from build123d import *

# Parameters (mm, degrees)
SKETCH1_W           = 68
SKETCH1_H           = 68
BOSS_EXTRUDE1_DEPTH = 10
SKETCH4_W           = 68
SKETCH4_H           = 68
SKETCH4_W_2         = 30
SKETCH4_H_2         = 30
BOSS_EXTRUDE3_DEPTH = 12
FILLET2_R           = 3
FILLET3_R           = 3
SKETCH5_R           = 3.25
CUT_EXTRUDE2_DEPTH  = 20
CHAMFER1_SIZE       = 3
CHAMFER2_SIZE       = 3


with BuildPart() as part:
    # Sketch1 → Boss-Extrude1 (new body)
    with BuildSketch(Plane(origin=(0, 0, 0), x_dir=(1, 0, 0), z_dir=(0, 1, 0))):
        Rectangle(SKETCH1_W, SKETCH1_H)
    extrude(amount=BOSS_EXTRUDE1_DEPTH)

    # Sketch4 → Boss-Extrude3 (add)
    with BuildSketch(Plane.XZ):
        Rectangle(SKETCH4_W, SKETCH4_H)
        Rectangle(SKETCH4_W_2, SKETCH4_H_2, mode=Mode.SUBTRACT)
    extrude(amount=BOSS_EXTRUDE3_DEPTH)

    # Fillet2
    fillet2_edges = [part.edges().sort_by_distance(p)[0] for p in [
        (34, -1, 34),
        (-34, -1, 34),
        (-34, -1, -34),
        (34, -1, -34),
    ]]
    fillet(fillet2_edges, radius=FILLET2_R)

    # Fillet3
    fillet3_edges = [part.edges().sort_by_distance(p)[0] for p in [
        (15, -6, 15),
        (-15, -6, 15),
        (-15, -6, -15),
        (15, -6, -15),
    ]]
    fillet(fillet3_edges, radius=FILLET3_R)

    # Sketch5 → Cut-Extrude2 (cut)
    with BuildSketch(Plane.XZ):
        with Locations(Location((0, 0, 0), (0, 0, 270))):
            Circle(SKETCH5_R)
    extrude(amount=-CUT_EXTRUDE2_DEPTH, mode=Mode.SUBTRACT)

    # Chamfer1
    chamfer1_edges = [part.edges().sort_by_distance(p)[0] for p in [
        (34, 10, 0),
        (0, 10, 34),
        (0, 10, -34),
        (-34, 10, 0),
        (-33.121320344, 10, -33.121320344),
        (33.121320344, 10, -33.121320344),
        (-33.121320344, 10, 33.121320344),
        (33.121320344, 10, 33.121320344),
    ]]
    chamfer(chamfer1_edges, length=CHAMFER1_SIZE - 0.0001)  # a hair under: the kernel refuses the full size

    # Chamfer2
    chamfer2_edges = [part.edges().sort_by_distance(p)[0] for p in [
        (0, 0, 15),
        (0, 0, -15),
        (15, 0, 0),
        (-15, 0, 0),
        (14.121320344, 0, 14.121320344),
        (14.121320344, 0, -14.121320344),
        (-14.121320344, 0, -14.121320344),
        (-14.121320344, 0, 14.121320344),
    ]]
    chamfer(chamfer2_edges, length=CHAMFER2_SIZE - 0.0001)  # a hair under: the kernel refuses the full size


solid = part.part
Model file for the job. Use its own axes, mm. A direction names the side the tool comes from. Give positions to 0.01 mm unless a question says otherwise; leave off trailing zeros. Write each loop counter-clockwise with the first axis right and the second up, starting at its lowest first coordinate (ties: lowest second). Pieces come first, ordered by that corner, then holes. Notation, with made-up numbers: (-9.75, 32.25) - (2.25, 32.25) arc R10 ccw to (2.25, 49.25) - close; hole circle Ø1 at (-27.75, 72). An arc over 180 degrees is marked (long way). Answer as CSV lines item,"result".
1. Band-saw the part on D-D (y = 8.25). Write the cut outline in (x, z), and give its area (3 significant figures).
Responses:
outline,"(-32.75, -31) arc R1.75 ccw to (-31, -32.75) - (31, -32.75) arc R1.75 ccw to (32.75, -31) - (32.75, 31) arc R1.75 ccw to (31, 32.75) - (-31, 32.75) arc R1.75 ccw to (-32.75, 31) - close; hole circle Ø6.5 at (0, 0)"
area,"4,250 mm2"
2. Drill centre lines: L1, parallel to X at y = 6.5, z = 0; L2, parallel to X at y = -6.25, z = 12. Where is each one in solid material? Low to high. Write a range as [from, to].
Responses:
L1,"x = [-34, -3.25], [3.25, 34]"
L2,"x = [-34, -15], [15, 34]"
3. Band-saw the part on C-C (x = -8). Write the cut outline in (y, z), and give its area (3 significant figures).
Responses:
outline,"(-12, -34) - (7, -34) - (10, -31) - (10, 31) - (7, 34) - (-12, 34) - (-12, 15) - (-3, 15) - (0, 12) - (0, -12) - (-3, -15) - (-12, -15) - close"
area,"1,140 mm2"
4. Pin check, flat tip, straight feed: pin 1 (7 mm diameter, centred on x = -5, z = -1, fed in from -Y). Stop position of the tip, or through.
Responses:
pin 1,"stops at y = 0"
5. 3-axis set-ups, long thin cutter, end or side, ignore diameter. For faces 1 (the face through (-13.06, -1.48, 13.03)), 2 (the face through (33.1, -2.63, -33.14)): which of +Z, -Z, +X, -X, +Y, -Y reach the whole face in a straight line?
Responses:
face 1,"-Y"
face 2,"-Z, +X, +Y, -Y"
6. Two-plate mould, pull along X, no slides. Class faces 3 (the face through (6, 10, 0)), 4 (the face through (-14.1, -7.56, 14.14)), 5 (the face through (-32.03, 8.52, -32.06)): +X half, -X half, draft (parallel to the pull), parting line (faces both ways), or undercut.
Responses:
face 3,"draft"
face 4,"undercut"
face 5,"-X half"
7. Band-saw the part on A-A (z = 0). Write the cut outline in (x, y), and give its area (3 significant figures).
Responses:
outline,"(-34, -12) - (-15, -12) - (-15, -3) - (-12, 0) - (-3.25, 0) - (-3.25, 10) - (-31, 10) - (-34, 7) - close; (3.25, 0) - (12, 0) - (15, -3) - (15, -12) - (34, -12) - (34, 7) - (31, 10) - (3.25, 10) - close"
area,"1,070 mm2"
8. Band-saw the part on B-B (y = -9). Write the cut outline in (x, z), and give its area (3 significant figures).
Responses:
outline,"(-34, -31) arc R3 ccw to (-31, -34) - (31, -34) arc R3 ccw to (34, -31) - (34, 31) arc R3 ccw to (31, 34) - (-31, 34) arc R3 ccw to (-34, 31) - close; hole (-15, -12) arc R3 ccw to (-12, -15) - (12, -15) arc R3 ccw to (15, -12) - (15, 12) arc R3 ccw to (12, 15) - (-12, 15) arc R3 ccw to (-15, 12) - close"
area,"3,720 mm2"
